Model file for the job. Use its own axes, mm. A direction names the side the tool comes from. Give positions to 0.01 mm unless a question says otherwise; leave off trailing zeros. Loops run counter-clockwise (first coordinate to the right, second up) from the corner with the lowest first, then second, coordinate; pieces in that order, holes last. Notation, with made-up numbers: M 46,4.25 L 100,4.25 A18 ccw 100,14.25 Z; hole C -7.5,21 d5. An arc over 180 degrees is marked long. Answer in a Markdown table with one row per item.
```python
from build123d import *

# Parameters (mm, degrees)
SKETCH1_W             = 120
SKETCH1_H             = 86
RAIL_PLATE_DEPTH      = 4
DOVETAIL_RAIL_DEPTH   = 40
BOLT_HOLES_DEPTH      = 75.491610266
BOLT_HOLES_DEPTH_BACK = 75.491610266
SKETCH3_R             = 1.7


with BuildPart() as part:
    # Sketch1 → Rail Plate (new body)
    with BuildSketch(Plane(origin=(0, 0, 0), x_dir=(1, 0, 0), z_dir=(0, 1, 0))):
        Rectangle(SKETCH1_W, SKETCH1_H)
    extrude(amount=RAIL_PLATE_DEPTH)

    # Sketch2 → Dovetail Rail (add, symmetric)
    with BuildSketch(Plane.XY):
        Polygon((-15, 3.5), (15, 3.5), (19, 10), (-19, 10), align=None)
    extrude(amount=DOVETAIL_RAIL_DEPTH, both=True)

    # Sketch3 → Bolt Holes (cut, two sides: drawn at the far end of the back side and taken through both)
    with BuildSketch(Plane(origin=(0, 0, 0), x_dir=(1, 0, 0), z_dir=(0, 1, 0)).offset(-BOLT_HOLES_DEPTH_BACK)):
        with Locations(Location((-40, -35, 0), (0, 0, 270))):
            Circle(SKETCH3_R)
        with Locations(Location((-40, 35, 0), (0, 0, 270))):
            Circle(SKETCH3_R)
        with Locations(Location((40, -35, 0), (0, 0, 270))):
            Circle(SKETCH3_R)
        with Locations(Location((40, 35, 0), (0, 0, 270))):
            Circle(SKETCH3_R)
        with Locations(Location((-52, -13, 0), (0, 0, 270))):
            Circle(SKETCH3_R)
        with Locations(Location((-52, 13, 0), (0, 0, 270))):
            Circle(SKETCH3_R)
        with Locations(Location((52, -13, 0), (0, 0, 270))):
            Circle(SKETCH3_R)
        with Locations(Location((52, 13, 0), (0, 0, 270))):
            Circle(SKETCH3_R)
    extrude(amount=BOLT_HOLES_DEPTH + BOLT_HOLES_DEPTH_BACK, mode=Mode.SUBTRACT)


solid = part.part
```
(1) Saw through at D-D, the plane x = -11.5. Give the cut face in (y, z), and give its area (3 significant figures).
Established:
| item | result |
|---|---|
| outline | M 0,-43 L 4,-43 L 4,-40 L 10,-40 L 10,40 L 4,40 L 4,43 L 0,43 Z |
| area | 824 mm2 |
(2) Saw through at B-B, the plane x = -52. Give the cut face in (y, z), and give its area (3 significant figures).
Established:
| item | result |
|---|---|
| outline | M 0,-43 L 4,-43 L 4,-14.7 L 0,-14.7 Z; M 0,-11.3 L 4,-11.3 L 4,11.3 L 0,11.3 Z; M 0,14.7 L 4,14.7 L 4,43 L 0,43 Z |
| area | 317 mm2 |
(3) Mould opens along Z. For faces 1 (the cylindrical face through (52.51, 1.97, -11.38)), 2 (the cylindrical face through (38.34, 1.97, 34.63)), 3 (the flat face through (-60, 2, 1)), 4 (the flat face through (-1, 2, 43)) say: pulls with the +Z half, pulls with the -Z half, needs draft (parallel to the pull), parting line crosses it, or undercut.
Established:
| item | result |
|---|---|
| face 1 | undercut |
| face 2 | undercut |
| face 3 | needs draft |
| face 4 | pulls with the +Z half |
(4) Flat gauge pins, fed straight in: P1, Ø1, axis at x = -38, z = 29, coming from the +Y side; P2, Ø2, axis at x = -52, z = -13, coming from the -Y side; P3, Ø5, axis at y = 7, z = 3, coming from the -X side; P4, Ø1.8, axis at x = -8.5, y = 7, coming from the +Z side. Where does each tip first touch, or does it go through?
Established:
| item | result |
|---|---|
| P1 | stops at y = 4 |
| P2 | passes through |
| P3 | stops at x = -18.69 |
| P4 | stops at z = 40 |
(5) Saw through at A-A, the plane z = 35. Give the cut face in (x, y).
Established:
| item | result |
|---|---|
| outline | M -60,0 L -41.7,0 L -41.7,4 L -60,4 Z; M -38.3,0 L 38.3,0 L 38.3,4 L 15.31,4 L 19,10 L -19,10 L -15.31,4 L -38.3,4 Z; M 41.7,0 L 60,0 L 60,4 L 41.7,4 Z |
(6) Which spindle directions (+Z, -Z, +X, -X, +Y, -Y) get a long thin tool onto all of the face, cutting with end or side? Do faces 5 (the flat face through (17.13, 6.96, 0.56)), 6 (the flat face through (-17.18, 7.04, 0.56)), 7 (the flat face through (0, 7, -40)), 8 (the flat face through (0, 7, 40)). Say none if no direction does.
Established:
| item | result |
|---|---|
| face 5 | +Z, -Z, +X |
| face 6 | +Z, -Z, -X |
| face 7 | -Z, +X, -X, +Y |
| face 8 | +Z, +X, -X, +Y |
(7) Saw through at C-C, the plane z = 24. Give the cut face in (x, y).
Established:
| item | result |
|---|---|
| outline | M -60,0 L 60,0 L 60,4 L 15.31,4 L 19,10 L -19,10 L -15.31,4 L -60,4 Z |
(8) Wall check: L1, parallel to X at y = 1.5, z = 35; L2, parallel to Z at x = -40, y = 0.95; L3, parallel to X at y = 1.9, z = 13. Give the ranges that are in metal, low to high.
Established:
| item | result |
|---|---|
| L1 | x = -60 to -41.7, -38.3 to 38.3, 41.7 to 60 |
| L2 | z = -43 to -36.7, -33.3 to 33.3, 36.7 to 43 |
| L3 | x = -60 to -53.7, -50.3 to 50.3, 53.7 to 60 |
